```python
from build123d import *

# Parameters (mm, degrees)
SKETCH1_R           = 2.38125
SKETCH1_W           = 3.2766
SKETCH1_H           = 3.2766
BOSS_EXTRUDE1_DEPTH = 4.7625


with BuildPart() as part:
    # Sketch1 → Boss-Extrude1 (new body)
    with BuildSketch(Plane.XY):
        with BuildLine():
            Line((0, 6.35), (76.2, 6.35))
            ThreePointArc((76.2, 6.35), (82.55, 0), (76.2, -6.35))
            Line((76.2, -6.35), (0, -6.35))
            ThreePointArc((0, -6.35), (-6.35, 0), (0, 6.35))
        make_face()
        with Locations(Location((0, 0, 0), (0, 0, 180))):
            Circle(SKETCH1_R, mode=Mode.SUBTRACT)
        with Locations((76.2, 0)):
            Rectangle(SKETCH1_W, SKETCH1_H, mode=Mode.SUBTRACT)
    extrude(amount=BOSS_EXTRUDE1_DEPTH)


solid = part.part
```
Check sheet for the modelled part. Datum: model origin and axes. Units: mm. A direction names the side the tool comes from. Round coordinates to 2 decimals unless told otherwise and drop trailing zeros. Loops run counter-clockwise (first coordinate to the right, second up) from the corner with the lowest first, then second, coordinate; pieces in that order, holes last. Notation, with made-up numbers: M 37,-33 L 63,-33 A5 cw 63,-26 Z; hole C -11,60 d8. An arc over 180 degrees is marked long. Answer as a JSON object with one key per item and string values.
1. Section check B-B (y = 0). Record the boundary of the cut face in (x, z).
Reply:
{"outline": "M -6.35,0 L -2.38,0 L -2.38,4.76 L -6.35,4.76 Z; M 2.38,0 L 74.56,0 L 74.56,4.76 L 2.38,4.76 Z; M 77.84,0 L 82.55,0 L 82.55,4.76 L 77.84,4.76 Z"}
2. Section check A-A (z = 1.7). Record the boundary of the cut face in (x, y), plus the area to 3 significant figures.
Reply:
{"outline": "M 0,-6.35 L 76.2,-6.35 A6.35 ccw 76.2,6.35 L 0,6.35 A6.35 ccw Z; hole C 0,0 d4.76; hole M 74.56,-1.64 L 77.84,-1.64 L 77.84,1.64 L 74.56,1.64 Z", "area": "1,070 mm²"}
3. Gauge pin test, flat end, axial feed: P1, Ø2, axis at y = -1.5, z = 2, coming from the +X side. Record the tip position at first contact, or that the pin passes through.
Reply:
{"P1": "stops at x = 82.53"}
4. Access from +Z, -Z, +X, -X, +Y, -Y to the whole of each face (thin tool, end or side, straight path). Record for faces 4 (the flat face through (76, 1.638, 2)), 5 (the flat face through (39, 0, 0)).
Reply:
{"face 4": "+Z, -Z", "face 5": "-Z, +X, -X, +Y, -Y"}
5. Mould release check, pull along Y, two halves, no side actions. Record for faces 1 (the flat face through (39, 0, 4.762)), 2 (the flat face through (74.562, 0, 2)), 3 (the flat face through (39, -6.35, 2)): pulls with the +Y half, pulls with the -Y half, needs draft (parallel to the pull), parting line crosses it, or undercut.
Reply:
{"face 1": "needs draft", "face 2": "undercut", "face 3": "pulls with the -Y half"}
6. Scan lines: line 1 (X direction, y = 0.5, z = 2); line 2 (Y direction, x = 0, z = 2.35); line 3 (X direction, y = -1, z = 1.05). Record each from-to range of solid material in increasing order.
Reply:
{"line 1": "x = -6.33 to -2.33, 2.33 to 74.56, 77.84 to 82.53", "line 2": "y = -6.35 to -2.38, 2.38 to 6.35", "line 3": "x = -6.27 to -2.16, 2.16 to 74.56, 77.84 to 82.47"}
